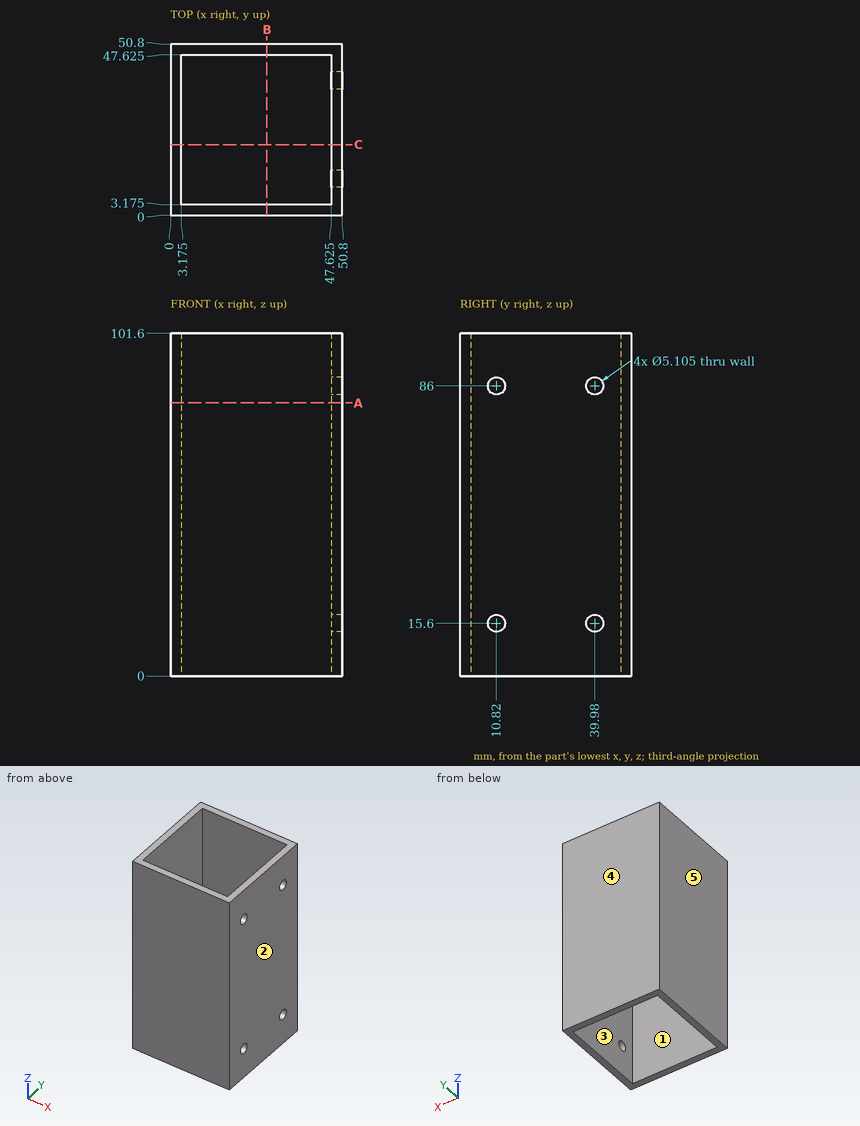
Input: dimensioned drawing with shaded views. Units: mm. Origin: part minimum x, y, z. A direction names the side the tool comes from. Give positions to 0.01 mm unless a question says otherwise; leave off trailing zeros. Loops run counter-clockwise (first coordinate to the right, second up) from the corner with the lowest first, then second, coordinate; pieces in that order, holes last. Notation, with made-up numbers: (48.5, -11.75) - (81.5, -11.75) arc R27 cw to (81.5, 21.25) - close; hole circle Ø5 at (-11, -31). An arc over 180 degrees is marked (long way). Answer as CSV lines item,"result". Start each with the question number.
(1) Section query A-A (z = 81). Output: boundary loops of the cut face in (x, y) (1 decimal).
(2) Ray query, line 1 along X through (y, z) = (30, 24.5) (1 decimal); line 2 along X through (y, z) = (9, 87.5) (1 decimal). Return the intervals inside material, ascending. Write a range as [from, to].
(3) Mould query, pull axis X, two halves, no side actions, for the marked faces 3, 4 and 5. Classes: +X half, -X half, draft (parallel to the pull), parting line (faces both ways), or undercut.
(4) Reachability of the marked faces 1 and 2 from +Z, -Z, +X, -X, +Y, -Y: full face, straight path, thin tool, end or side. Return the list, or none.
(5) Pin query (flat end, axial travel): P1, Ø8, axis at x = 9, y = 27, coming from the -Z side; P2, Ø3, axis at y = 10.82, z = 86, coming from the +X side (3 decimals). Return the tip coordinate at first contact, or that it passes through.
(6) Section query B-B (x = 28.5). Output: boundary loops of the cut face in (y, z) (1 decimal).
Worked answers:
1,outline,"(0, 0) - (50.8, 0) - (50.8, 50.8) - (0, 50.8) - close; hole (3.2, 3.2) - (47.6, 3.2) - (47.6, 47.6) - (3.2, 47.6) - close"
2,line 1,"x = [0, 3.2], [47.6, 50.8]"
2,line 2,"x = [0, 3.2]"
3,face 3,"undercut"
3,face 4,"draft"
3,face 5,"-X half"
4,face 1,"+Z, -Z"
4,face 2,"+Z, -Z, +X, +Y, -Y"
5,P1,"passes through"
5,P2,"stops at x = 3.175"
6,outline,"(0, 0) - (3.2, 0) - (3.2, 101.6) - (0, 101.6) - close; (47.6, 0) - (50.8, 0) - (50.8, 101.6) - (47.6, 101.6) - close"
